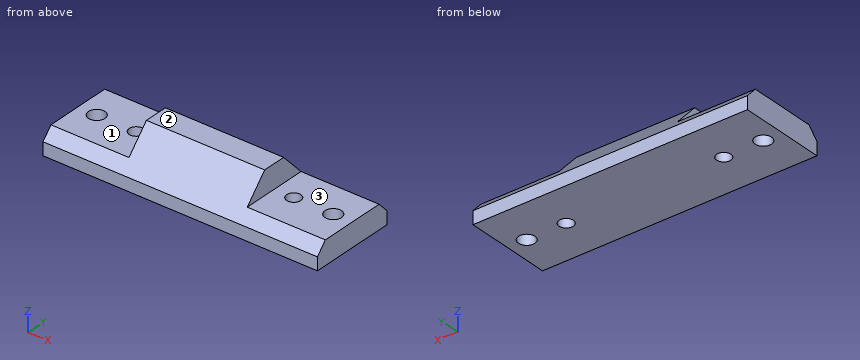
```python
from build123d import *

# Parameters (mm, degrees)
F0_W          = 38
F0_H          = 18.5
F0_R          = 1.5
F0_W_2        = 10
F0_R_2        = 1.75
F1_DEPTH      = 10
F3_DEPTH      = 58.001
F4_W          = 16.5
F4_H          = 12
F5_DEPTH      = 25
F5_DEPTH_BACK = 25


with BuildPart() as f1:
    # F0 (on Top) → F1 (new body)
    with BuildSketch(Plane.XY):
        Rectangle(F0_W, F0_H)
        with Locations((-16.65, 0)):
            Circle(F0_R, mode=Mode.SUBTRACT)
        with Locations((16.65, 0)):
            Circle(F0_R, mode=Mode.SUBTRACT)
        with Locations((24, 0)):
            Rectangle(F0_W_2, F0_H)
        with Locations((25, 0)):
            Circle(F0_R_2, mode=Mode.SUBTRACT)
        with Locations((-24, 0)):
            Rectangle(F0_W_2, F0_H)
        with Locations((-25, 0)):
            Circle(F0_R_2, mode=Mode.SUBTRACT)
    extrude(amount=F1_DEPTH)

    # F2 (on face) → F3 (cut, through all)
    with BuildSketch(Plane.YZ.offset(29)):
        Polygon((-9.25, 10), (-9.25, 2.72), (-4.625, 7.72), (-2.516, 10), align=None)
        Polygon((2.516, 10), (4.625, 7.72), (9.25, 2.72), (9.25, 10), align=None)
    extrude(amount=-F3_DEPTH, mode=Mode.SUBTRACT)

    # F4 (on Front) → F5 (cut, two sides)
    with BuildSketch(Plane.XZ) as f5_sk:
        with Locations((-20.75, 11)):
            Rectangle(F4_W, F4_H)
        with Locations((20.75, 11)):
            Rectangle(F4_W, F4_H)
    extrude(amount=F5_DEPTH, mode=Mode.SUBTRACT)
    extrude(f5_sk.sketch, amount=-F5_DEPTH_BACK, mode=Mode.SUBTRACT)


solid = f1.part
```
Verification items for the finished model (mm, model axes). Face numbers are marked on the shaded views. A direction names the side the tool comes from. Coordinates: 2 decimals unless noted, no trailing zeros. Order: outer loops, then holes, each group sorted by start corner. A loop starts at its lowest first (then second) coordinate and runs counter-clockwise, first axis right, second up. Notation, with made-up numbers: (51, 9.25) -> (79, 9.25) arc R29 cw to (79, 42.25) -> close; hole circle Ø11 at (-29.5, -3). An arc over 180 degrees is marked (long way). Put each result on its own line as item: value. Start each with the question number.
1) Cross-section at C-C (z = 2). Enter the section's corners in (x, y), plus the area to 3 significant figures.
2) Tool access check on the marked faces 1, 2 and 3. Record the directions out of +Z, -Z, +X, -X, +Y, -Y that give a thin tool (end or side, any length) a straight path to the whole face; none if there is none.
3) Material ranges on L1, parallel to Y at x = -16.65, z = 1.65; L2, parallel to Y at x = 25, z = 1.45; L3, parallel to Z at x = 24, y = -2.25, recorded low to high.
4) Go/stop test with flat-tipped pins: pin 1 (6 mm diameter, centred on y = 4, z = 6, fed in from +X); pin 2 (2.5 mm diameter, centred on y = 1.5, z = 7.5, fed in from -X); pin 3 (1 mm diameter, centred on x = -9, z = 3.5, fed in from +Y). Record where each tip stops, or that it passes through.
5) Cross-section at A-A (x = -25). Enter the section's corners in (y, z).
6) Cross-section at D-D (x = 14.5). Enter the section's corners in (y, z).
7) Cross-section at B-B (y = 0). Enter the section's corners in (x, z), plus the area to 3 significant figures.
Geometry check:
1. outline: (-29, -9.25) -> (29, -9.25) -> (29, 9.25) -> (-29, 9.25) -> close; hole circle Ø3.5 at (-25, 0); hole circle Ø3 at (-16.65, 0); hole circle Ø3 at (16.65, 0); hole circle Ø3.5 at (25, 0)
1. area: 1,040 mm^2
2. face 1: +Z, -X, +Y, -Y
2. face 2: +Z, +X, -X, +Y, -Y
2. face 3: +Z, +X, +Y, -Y
3. L1: y = -9.25 to -1.5, 1.5 to 9.25
3. L2: y = -9.25 to -1.75, 1.75 to 9.25
3. L3: z = 0 to 5
4. pin 1: stops at x = 29
4. pin 2: stops at x = -12.5
4. pin 3: stops at y = 8.99
5. outline: (-9.25, 0) -> (-1.75, 0) -> (-1.75, 5) -> (-7.14, 5) -> (-9.25, 2.72) -> close; (1.75, 0) -> (9.25, 0) -> (9.25, 2.72) -> (7.14, 5) -> (1.75, 5) -> close
6. outline: (-9.25, 0) -> (9.25, 0) -> (9.25, 2.72) -> (7.14, 5) -> (-7.14, 5) -> (-9.25, 2.72) -> close
7. outline: (-29, 0) -> (-26.75, 0) -> (-26.75, 5) -> (-29, 5) -> close; (-23.25, 0) -> (-18.15, 0) -> (-18.15, 5) -> (-23.25, 5) -> close; (-15.15, 0) -> (15.15, 0) -> (15.15, 5) -> (12.5, 5) -> (12.5, 10) -> (-12.5, 10) -> (-12.5, 5) -> (-15.15, 5) -> close; (18.15, 0) -> (23.25, 0) -> (23.25, 5) -> (18.15, 5) -> close; (26.75, 0) -> (29, 0) -> (29, 5) -> (26.75, 5) -> close
7. area: 350 mm^2
